The listing builds one solid part. Answer for the finished solid, in the listing's coordinates (mm). Give positions to 0.01 mm unless a question says otherwise; leave off trailing zeros. Order: outer loops, then holes, each group sorted by start corner. A loop starts at its lowest first (then second) coordinate and runs counter-clockwise, first axis right, second up.
```python
from build123d import *

# Parameters (mm, degrees)
SKETCH1_R           = 1.75
BOSS_EXTRUDE2_DEPTH = 3


with BuildPart() as part:
    # Sketch1 → Boss-Extrude2 (new body)
    with BuildSketch(Plane.XY):
        with BuildLine():
            Line((12, 55), (0, 55))
            Line((0, 55), (-12, 55))
            Line((-12, 55), (-12, 69.5))
            Line((-12, 69.5), (-12, 74.033776076))
            ThreePointArc((-12, 74.033776076), (-28.701257427, 69.290964938), (-43.864503726, 60.835066474))
            Line((-43.864503726, 60.835066474), (-30.405591591, 47.376154339))
            Line((-30.405591591, 47.376154339), (-47.376154339, 30.405591591))
            Line((-47.376154339, 30.405591591), (-60.835066474, 43.864503726))
            ThreePointArc((-60.835066474, 43.864503726), (-69.290964938, 28.701257427), (-74.033776076, 12))
            Line((-74.033776076, 12), (-55, 12))
            Line((-55, 12), (-55, -12))
            Line((-55, -12), (-74.033776076, -12))
            ThreePointArc((-74.033776076, -12), (-69.290964938, -28.701257427), (-60.835066474, -43.864503726))
            Line((-60.835066474, -43.864503726), (-47.376154339, -30.405591591))
            Line((-47.376154339, -30.405591591), (-30.405591591, -47.376154339))
            Line((-30.405591591, -47.376154339), (-43.864503726, -60.835066474))
            ThreePointArc((-43.864503726, -60.835066474), (-28.701257427, -69.290964938), (-12, -74.033776076))
            Line((-12, -74.033776076), (-12, -55))
            Line((-12, -55), (12, -55))
            Line((12, -55), (12, -74.033776076))
            ThreePointArc((12, -74.033776076), (28.701257427, -69.290964938), (43.864503726, -60.835066474))
            Line((43.864503726, -60.835066474), (30.405591591, -47.376154339))
            Line((30.405591591, -47.376154339), (47.37615434, -30.405591591))
            Line((47.37615434, -30.405591591), (60.835066474, -43.864503726))
            ThreePointArc((60.835066474, -43.864503726), (69.290964938, -28.701257427), (74.033776076, -12))
            Line((74.033776076, -12), (55, -12))
            Line((55, -12), (55, 12))
            Line((55, 12), (74.033776076, 12))
            ThreePointArc((74.033776076, 12), (69.290964938, 28.701257427), (60.835066474, 43.864503726))
            Line((60.835066474, 43.864503726), (47.376154339, 30.405591591))
            Line((47.376154339, 30.405591591), (30.405591591, 47.37615434))
            Line((30.405591591, 47.37615434), (43.864503726, 60.835066474))
            ThreePointArc((43.864503726, 60.835066474), (28.701257427, 69.290964938), (12, 74.033776076))
            Line((12, 74.033776076), (12, 69.5))
            Line((12, 69.5), (12, 55))
        make_face()
        with Locations((-37.123106012, -61.164736573)):
            Circle(SKETCH1_R, mode=Mode.SUBTRACT)
        with Locations((-17, -69.5)):
            Circle(SKETCH1_R, mode=Mode.SUBTRACT)
        with Locations((-61.164736573, -37.123106012)):
            Circle(SKETCH1_R, mode=Mode.SUBTRACT)
        with Locations((-69.5, -17)):
            Circle(SKETCH1_R, mode=Mode.SUBTRACT)
        with Locations((17, -69.5)):
            Circle(SKETCH1_R, mode=Mode.SUBTRACT)
        with Locations((37.123106012, -61.164736573)):
            Circle(SKETCH1_R, mode=Mode.SUBTRACT)
        with Locations((61.164736573, -37.123106012)):
            Circle(SKETCH1_R, mode=Mode.SUBTRACT)
        with Locations((69.5, -17)):
            Circle(SKETCH1_R, mode=Mode.SUBTRACT)
        with Locations((-69.5, 17)):
            Circle(SKETCH1_R, mode=Mode.SUBTRACT)
        with Locations((-61.164736573, 37.123106012)):
            Circle(SKETCH1_R, mode=Mode.SUBTRACT)
        with Locations((-37.123106012, 61.164736573)):
            Circle(SKETCH1_R, mode=Mode.SUBTRACT)
        with Locations((-17, 69.5)):
            Circle(SKETCH1_R, mode=Mode.SUBTRACT)
        with Locations((69.5, 17)):
            Circle(SKETCH1_R, mode=Mode.SUBTRACT)
        with Locations((61.164736573, 37.123106012)):
            Circle(SKETCH1_R, mode=Mode.SUBTRACT)
        with BuildLine():
            ThreePointArc((18.75, 69.5), (17, 67.75), (15.25, 69.5))
            ThreePointArc((15.25, 69.5), (17, 71.25), (18.75, 69.5))
        make_face(mode=Mode.SUBTRACT)
        with Locations((37.123106012, 61.164736573)):
            Circle(SKETCH1_R, mode=Mode.SUBTRACT)
    extrude(amount=BOSS_EXTRUDE2_DEPTH)


solid = part.part
```
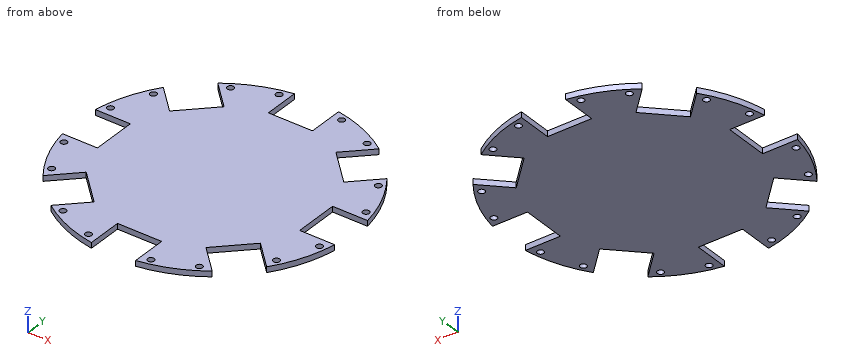
1) Given P1, Ø1.5, axis at x = -3, z = 1.5, coming from the +Y side; P2, Ø1, axis at y = -8.5, z = 2, coming from the -X side; P3, Ø0.9, axis at y = -1.5, z = 1, coming from the +X side, each flat-ended and moving along its own axis, determine where each tip first touches the part or whether it passes through.
Geometry says:
P1: stops at y = 55
P2: stops at x = -55
P3: stops at x = 55
2) Straight lines are drawn through the part: probe 1 along Y at (x, z) = (17, 2.4); probe 2 along Y at (x, z) = (-31, 1.2); probe 3 along X at (y, z) = (39.5, 0.65). For each, find the intervals that lie inside material, in ascending order.
Geometry says:
probe 1: y = -73.05 to -71.25, -67.75 to 67.75, 71.25 to 73.05
probe 2: y = -68.29 to -47.97, -46.78 to 46.78, 47.97 to 68.29
probe 3: x = -63.76 to -56.47, -38.28 to 38.28, 56.47 to 63.76
3) Find section C-C (x = 69.5). Write down the section's boundary in (y, z), then the cut area to 3 significant figures.
Geometry says:
outline: (-28.19, 0) - (-18.75, 0) - (-18.75, 3) - (-28.19, 3) - close; (-15.25, 0) - (-12, 0) - (-12, 3) - (-15.25, 3) - close; (12, 0) - (15.25, 0) - (15.25, 3) - (12, 3) - close; (18.75, 0) - (28.19, 0) - (28.19, 3) - (18.75, 3) - close
area: 76.1 mm2
4) Find section A-A (x = -17). Write down the section's boundary in (y, z).
Geometry says:
outline: (-73.05, 0) - (-71.25, 0) - (-71.25, 3) - (-73.05, 3) - close; (-67.75, 0) - (67.75, 0) - (67.75, 3) - (-67.75, 3) - close; (71.25, 0) - (73.05, 0) - (73.05, 3) - (71.25, 3) - close
